Can you work these out from the drawing? Everything is in mm from the part's minimum corner. Round coordinates to 2 decimals unless told otherwise and drop trailing zeros. Write each loop counter-clockwise with the first axis right and the second up, starting at its lowest first coordinate (ties: lowest second). Pieces come first, ordered by that corner, then holes. Notation, with made-up numbers: M -37,88.25 L -13,88.25 A36 ccw -13,123.25 Z; hole C 14,12.25 d2. An arc over 180 degrees is marked long. Answer in a Markdown table with one row per item. Add a question column.
(1) Suppose I cut it at D-D, the plane y = 16. Write out the boundary of the cut face in (x, z), then the cut area to 3 significant figures.
(2) I'm going to push flat-ended pins straight in: pin 1 (5 mm diameter, centred on x = 19.5, z = 7, fed in from -Y); pin 2 (1 mm diameter, centred on x = 36.5, z = 26.5, fed in from +Y); pin 3 (3 mm diameter, centred on y = 34, z = 6, fed in from +X); pin 4 (8 mm diameter, centred on x = 37, y = 27.5, fed in from -Z). Where does each tip first touch, or does it pass through?
(3) If I drill on probe 1 along Y at (x, z) = (27, 29.5); probe 2 along Y at (x, z) = (27, 6); probe 3 along Z at (x, y) = (37, 5), over which ranges is the centre line in solid material (lowest first)?
(4) Suppose I cut it at C-C, the plane z = 16.5. Write out the boundary of the cut face in (x, y).
(5) If we mould it in two halves opening along X, with no side actions, what happens to the marked faces 1, 2 and 3? For each: released by +X, released by -X, zero draft, split by the parting line, or undercut.
(6) Suppose I cut it at B-B, the plane x = 22. Write out the boundary of the cut face in (y, z), then the cut area to 3 significant figures.
(7) Suppose I cut it at A-A, the plane y = 27. Write out the boundary of the cut face in (x, z), then the cut area to 4 significant figures.
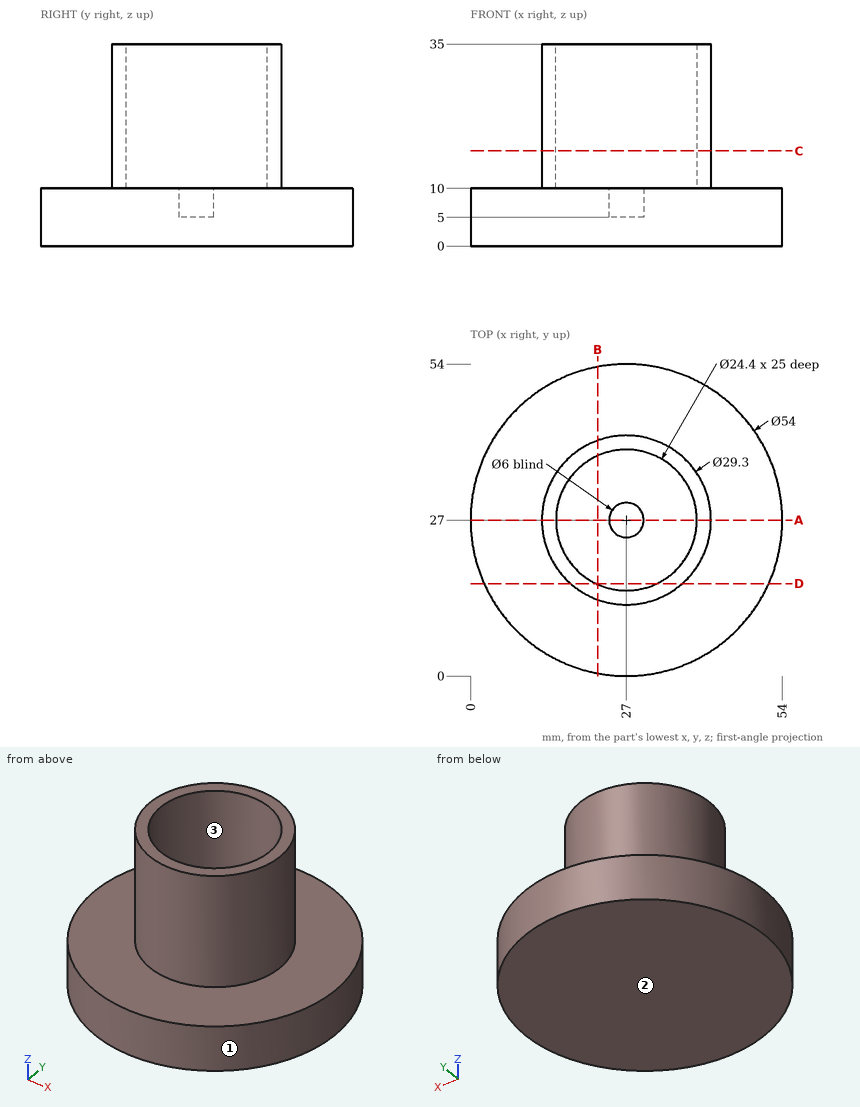
Calculated:
| question | item | result |
|---|---|---|
| 1 | outline | M 2.34,0 L 51.66,0 L 51.66,10 L 36.68,10 L 36.68,35 L 32.28,35 L 32.28,10 L 21.72,10 L 21.72,35 L 17.32,35 L 17.32,10 L 2.34,10 Z |
| 1 | area | 713 mm² |
| 2 | pin 1 | y = 0.47 |
| 2 | pin 2 | y = 38.56 |
| 2 | pin 3 | x = 53.43 |
| 2 | pin 4 | z = 0 |
| 3 | probe 1 | 12.35 to 14.8, 39.2 to 41.65 |
| 3 | probe 2 | 0 to 24, 30 to 54 |
| 3 | probe 3 | 0 to 10 |
| 4 | outline | C 27,27 d29.3; hole C 27,27 d24.4 |
| 5 | face 1 | split by the parting line |
| 5 | face 2 | zero draft |
| 5 | face 3 | undercut |
| 6 | outline | M 0.47,0 L 53.53,0 L 53.53,10 L 40.77,10 L 40.77,35 L 38.13,35 L 38.13,10 L 15.87,10 L 15.87,35 L 13.23,35 L 13.23,10 L 0.47,10 Z |
| 6 | area | 663 mm² |
| 7 | outline | M 0,0 L 54,0 L 54,10 L 41.65,10 L 41.65,35 L 39.2,35 L 39.2,10 L 30,10 L 30,5 L 24,5 L 24,10 L 14.8,10 L 14.8,35 L 12.35,35 L 12.35,10 L 0,10 Z |
| 7 | area | 632.5 mm² |
